from build123d import *

# Parameters (mm, degrees)
SKETCH1_R           = 2.5
BOSS_EXTRUDE1_DEPTH = 12
CUT_EXTRUDE2_DEPTH  = 5
SKETCH2_R           = 20.406966807
SKETCH2_R_2         = 17.406966807
CUT_EXTRUDE1_DEPTH  = 5
SKETCH4_W           = 285.875648179
SKETCH4_H           = 19.682926892
CUT_EXTRUDE3_DEPTH  = 147.5


with BuildPart() as part:
    # Sketch1 → Boss-Extrude1 (new body)
    with BuildSketch(Plane.XY):
        with BuildLine():
            Line((-26.955627075, 25.359398414), (44.050751749, 70.198338512))
            add(Edge.make_bspline(
                [(44.050751749, 70.198338512), (62.087157858, 60.129124735), (102.236821697, -14.309839041), (30.255220871, -56.610877482)],
                knots=[0, 0, 0, 0, 1, 1, 1, 1], degree=3))
            Line((30.255220871, -56.610877482), (-92.542495842, -130.724182913))
            Line((-92.542495842, -130.724182913), (-109.546280871, -97.192243206))
            Line((-109.546280871, -97.192243206), (-53.551819625, -58.475967995))
            ThreePointArc((-53.551819625, -58.475967995), (-44.950344781, -47.729789478), (-43.667906214, -34.025006607))
            Line((-43.667906214, -34.025006607), (-55.484471769, 25.012678553))
            ThreePointArc((-55.484471769, 25.012678553), (-55.229156607, 26.186005417), (-54.194896814, 26.796077907))
            Line((-54.194896814, 26.796077907), (-36.765460017, 28.917713338))
            Line((-36.765460017, 28.917713338), (-34.712668517, 26.525380142))
            ThreePointArc((-34.712668517, 26.525380142), (-31.051074716, 24.4992182), (-26.955627075, 25.359398414))
        make_face()
        Circle(SKETCH1_R, mode=Mode.SUBTRACT)
        with BuildLine():
            Line((38.077539086, 8.627342387), (31.457970773, 37.843392922))
            ThreePointArc((31.457970773, 37.843392922), (36.113405951, 45.226418252), (43.49643128, 40.570983074))
            Line((43.49643128, 40.570983074), (50.115999593, 11.354932539))
            ThreePointArc((50.115999593, 11.354932539), (47.829544092, -18.785170217), (28.993629861, -42.425432651))
            Line((28.993629861, -42.425432651), (-1.139071825, -63.018184329))
            ThreePointArc((-1.139071825, -63.018184329), (-9.716926906, -61.404944758), (-8.103687335, -52.827089677))
            Line((-8.103687335, -52.827089677), (22.029014352, -32.234337999))
            ThreePointArc((22.029014352, -32.234337999), (36.340317452, -14.272748403), (38.077539086, 8.627342387))
        make_face(mode=Mode.SUBTRACT)
    boss_extrude1 = extrude(amount=-BOSS_EXTRUDE1_DEPTH)

    # Sketch3 → Cut-Extrude2 (cut)
    with BuildSketch(Plane(origin=(0, 0, -12), x_dir=(-1, 0, 0), z_dir=(0, 0, -1))):
        with BuildLine():
            Line((108.633361408, -98.992545924), (93.449492386, -128.935560359))
            Line((93.449492386, -128.935560359), (91.732523821, -127.89930155))
            Line((91.732523821, -127.89930155), (-29.231808811, -54.892516323))
            add(Edge.make_bspline(
                [(-44.065734477, 67.842412696), (-44.711989199, 67.409412256), (-45.319058391, 66.940521732), (-46.487121265, 65.960540056), (-47.04734625, 65.448744854), (-48.676831708, 63.866474713), (-49.695652132, 62.74980166), (-51.643061578, 60.433812481), (-52.570637695, 59.233568633), (-54.351661803, 56.76518688), (-55.206220539, 55.494184071), (-57.642169465, 51.637395526), (-59.108475151, 48.994377471), (-61.772216068, 43.585851359), (-62.968525898, 40.819830599), (-64.562191776, 36.579321004), (-65.059713989, 35.150465126), (-65.753925807, 32.983458962), (-65.976639631, 32.257164595), (-66.404295719, 30.796479627), (-66.609516748, 30.060994816), (-67.585549406, 26.379930292), (-68.207997329, 23.421535241), (-69.124162601, 17.476634327), (-69.417856055, 14.49012642), (-69.647875237, 8.486550939), (-69.584312973, 5.469492942), (-69.186185446, 0.918013899), (-69.001954276, -0.606436507), (-68.53395704, -3.614530288), (-68.249900615, -5.10403396), (-67.246805131, -9.528696616), (-66.377032654, -12.420063251), (-64.763908669, -16.667495261), (-64.174739481, -18.06835499), (-63.212508348, -20.146844678), (-62.87805617, -20.837039742), (-62.187699389, -22.200245629), (-61.831475952, -22.874060854), (-59.996492333, -26.20515645), (-58.3564207, -28.748698204), (-54.76187252, -33.614098874), (-52.807325031, -35.935907769), (-49.657387027, -39.264829798), (-48.576129174, -40.343226595), (-46.36681057, -42.431345516), (-45.23699415, -43.442927339), (-39.471767159, -48.350894333), (-34.491238963, -51.801735421), (-29.231808811, -54.892516323)],
                knots=[0, 0, 0, 0, 0.015625, 0.015625, 0.03125, 0.03125, 0.0625, 0.0625, 0.09375, 0.09375, 0.125, 0.125, 0.1875, 0.1875, 0.25, 0.25, 0.28125, 0.28125, 0.296875, 0.296875, 0.3125, 0.3125, 0.375, 0.375, 0.4375, 0.4375, 0.5, 0.5, 0.53125, 0.53125, 0.5625, 0.5625, 0.625, 0.625, 0.65625, 0.65625, 0.671875, 0.671875, 0.6875, 0.6875, 0.75, 0.75, 0.8125, 0.8125, 0.84375, 0.84375, 0.875, 0.875, 1, 1, 1, 1], degree=3))
            Line((-44.065734477, 67.842412696), (25.887763568, 23.668343261))
            ThreePointArc((25.887763568, 23.668343261), (31.348360423, 22.521436309), (36.230485491, 25.222985565))
            Line((36.230485491, 25.222985565), (37.586279366, 26.80303434))
            Line((37.586279366, 26.80303434), (53.417437888, 24.875952746))
            Line((53.417437888, 24.875952746), (41.706802558, -33.632485968))
            ThreePointArc((41.706802558, -33.632485968), (43.096111006, -48.479334078), (52.414375421, -60.121027471))
            Line((52.414375421, -60.121027471), (106.973050581, -97.844556472))
            Line((106.973050581, -97.844556472), (108.633361408, -98.992545924))
        make_face()
    cut_extrude2 = extrude(amount=-CUT_EXTRUDE2_DEPTH, mode=Mode.SUBTRACT)

    # Sketch2 → Cut-Extrude1 (cut)
    with BuildSketch(Plane(origin=(0, 0, -7), x_dir=(-1, 0, 0), z_dir=(0, 0, -1))):
        Circle(SKETCH2_R)
        Circle(SKETCH2_R_2, mode=Mode.SUBTRACT)
    cut_extrude1 = extrude(amount=-CUT_EXTRUDE1_DEPTH, mode=Mode.SUBTRACT)

    # Mirror2: Boss-Extrude1, Cut-Extrude2, Cut-Extrude1 across plane
    add(boss_extrude1.mirror(Plane.XY))
    add(cut_extrude2.mirror(Plane.XY), mode=Mode.SUBTRACT)
    add(cut_extrude1.mirror(Plane.XY), mode=Mode.SUBTRACT)

    # Sketch4 → Cut-Extrude3 (cut, symmetric)
    with BuildSketch(Plane(origin=(0, 0, 0), x_dir=(1, 0, 0), z_dir=(0, 1, 0))):
        with Locations((-41.859921239, 9.841463446)):
            Rectangle(SKETCH4_W, SKETCH4_H)
    extrude(amount=CUT_EXTRUDE3_DEPTH, both=True, mode=Mode.SUBTRACT)


solid = part.part
Verification items for the finished model (mm, model axes). A direction names the side the tool comes from. Coordinates: 2 decimals unless noted, no trailing zeros. Order: outer loops, then holes, each group sorted by start corner. A loop starts at its lowest first (then second) coordinate and runs counter-clockwise, first axis right, second up.
Item 1: Access from +Z, -Z, +X, -X, +Y, -Y to the whole of each face (thin tool, end or side, straight path). Record for faces 4 (the face through (6.752, -42.675, 3.451)), 5 (the face through (-45.391, 25.853, 9.535)), 6 (the face through (-100.925, -114.193, 3.249)).
Filled in:
face 4: +Z, -Z
face 5: +Z
face 6: +Z, -Z, -X, -Y
Item 2: Depth check by flat-ended pin: pin 1 (4 mm diameter, centred on x = 49, y = 1.5, fed in from -Z); pin 2 (8 mm diameter, centred on x = 0, y = 0, fed in from +Z); pin 3 (4 mm diameter, centred on x = 19.5, z = 9, fed in from -Y); pin 4 (3 mm diameter, centred on y = -56.5, z = 10, fed in from +X). Enter the tip coordinate at first touch or a pass-through.
Filled in:
pin 1: passes through
pin 2: stops at z = 7
pin 3: stops at y = -64.31
pin 4: stops at x = 32.92
Item 3: Material ranges on L1, parallel to Y at x = 0, z = 4.75; L2, parallel to Z at x = 45.5, y = 43.5; L3, parallel to Y at x = 6.5, z = 7.75, recorded low to high.
Filled in:
L1: y = -74.87 to -62.24, -47.29 to -20.41, -17.41 to -2.5, 2.5 to 17.41, 20.41 to 42.38
L2: z = 0 to 7
L3: y = -70.95 to -68.61, 44.12 to 46.49
Item 4: Section check A-A, the plane x = 10. Enter the section's corners in (y, z) (3 decimals).
Filled in:
outline: (-68.836, 0) - (-55.406, 0) - (-55.406, 7) - (-66.5, 7) - (-66.5, 12) - (-68.836, 12) - close; (-40.455, 0) - (48.696, 0) - (48.696, 12) - (46.331, 12) - (46.331, 7) - (17.789, 7) - (17.789, 2) - (14.248, 2) - (14.248, 7) - (-14.248, 7) - (-14.248, 2) - (-17.789, 2) - (-17.789, 7) - (-40.455, 7) - close
Item 5: Section check B-B, the plane y = -82. Enter the section's corners in (x, z), then the cut area to 3 significant figures.
Filled in:
outline: (-87.57, 0) - (-11.81, 0) - (-11.81, 12) - (-15.68, 12) - (-15.68, 7) - (-84.06, 7) - (-84.06, 12) - (-87.57, 12) - close
area: 567 mm2
Item 6: Release check for a two-part mould opening along X. For faces 1 (the face through (46.76, 26.17, 3.45)), 2 (the face through (-45.024, -47.911, 5.916)), 3 (the face through (-30.284, -93.149, 5.916)) record: +X half, -X half, draft (parallel to the pull), parting line (faces both ways), or undercut.
Filled in:
face 1: undercut
face 2: -X half
face 3: +X half
Item 7: Section check C-C, the plane y = 0. Give the number of separate pieces and of enclosed holes in the cut face, then the cut area to 3 significant figures.
Filled in:
separate pieces: 3
enclosed holes: 0
area: 720 mm2
